Read the model definition and answer for the solid it produces. Units are mm, in the model's axes. A direction names the side the tool comes from. Give positions to 0.01 mm unless a question says otherwise; leave off trailing zeros. Loops run counter-clockwise (first coordinate to the right, second up) from the corner with the lowest first, then second, coordinate; pieces in that order, holes last. Notation, with made-up numbers: (38, 87) -> (94, 87) arc R13 cw to (94, 103) -> close; hole circle Ø11 at (-29.5, 3). An arc over 180 degrees is marked (long way). Return JSON: item names as keys, results as strings. Group by question number.
Autodesk Inventor part; units mm, degrees
ref_plane "YZ Plane" through (0, 0, 0) normal (1, 0, 0) x (0, 1, 0)
ref_plane "XZ Plane" through (0, 0, 0) normal (0, 1, 0) x (-1, 0, 0)
ref_plane "XY Plane" through (0, 0, 0) normal (0, 0, 1) x (1, 0, 0)
sketch "Sketch1" plane through (0, 0, 0) normal (1, 0, 0) x (0, 1, 0)
  arc A0 (-4.3875, 5.1282) -> (-5.1282, 4.3875) centre (0, 0) ccw
  arc A1 (-5.1895, 7.3532) -> (-4.3875, 5.1282) centre (-1.9912, 7.249) ccw
  arc A2 (-3.0589, 6.016) -> (-4.8075, 7.6084) centre (-5.9352, 4.6137) ccw
  arc A3 (-4.8075, 7.6084) -> (-5.1895, 7.3532) centre (0, 0) ccw
  arc A4 (-2.091, 6.4169) -> (-3.0589, 6.016) centre (0, 0) ccw
  arc A5 (-1.9805, 8.7794) -> (-2.091, 6.4169) centre (0.9345, 7.4592) ccw
  arc A6 (-1.5299, 8.869) -> (-1.9805, 8.7794) centre (0, 0) ccw
  arc A7 (-0.5238, 6.7286) -> (-1.5299, 8.869) centre (-3.7179, 6.5338) ccw
  arc A8 (0.5238, 6.7286) -> (-0.5238, 6.7286) centre (0, 0) ccw
  arc A9 (1.5299, 8.869) -> (0.5238, 6.7286) centre (3.7179, 6.5338) ccw
  arc A10 (1.9805, 8.7794) -> (1.5299, 8.869) centre (0, 0) ccw
  arc A11 (2.091, 6.4169) -> (1.9805, 8.7794) centre (-0.9345, 7.4592) ccw
  arc A12 (3.0589, 6.016) -> (2.091, 6.4169) centre (0, 0) ccw
  arc A13 (4.8075, 7.6084) -> (3.0589, 6.016) centre (5.9352, 4.6137) ccw
  arc A14 (5.1895, 7.3532) -> (4.8075, 7.6084) centre (0, 0) ccw
  arc A15 (4.3875, 5.1282) -> (5.1895, 7.3532) centre (1.9912, 7.249) ccw
  arc A16 (5.1282, 4.3875) -> (4.3875, 5.1282) centre (0, 0) ccw
  arc A17 (7.3532, 5.1895) -> (5.1282, 4.3875) centre (7.249, 1.9912) ccw
  arc A18 (7.6084, 4.8075) -> (7.3532, 5.1895) centre (0, 0) ccw
  arc A19 (6.016, 3.0589) -> (7.6084, 4.8075) centre (4.6137, 5.9352) ccw
  arc A20 (6.4169, 2.091) -> (6.016, 3.0589) centre (0, 0) ccw
  arc A21 (8.7794, 1.9805) -> (6.4169, 2.091) centre (7.4592, -0.9345) ccw
  arc A22 (8.869, 1.5299) -> (8.7794, 1.9805) centre (0, 0) ccw
  arc A23 (6.7286, 0.5238) -> (8.869, 1.5299) centre (6.5338, 3.7179) ccw
  arc A24 (6.7286, -0.5238) -> (6.7286, 0.5238) centre (0, 0) ccw
  arc A25 (8.869, -1.5299) -> (6.7286, -0.5238) centre (6.5338, -3.7179) ccw
  arc A26 (8.7794, -1.9805) -> (8.869, -1.5299) centre (0, 0) ccw
  arc A27 (6.4169, -2.091) -> (8.7794, -1.9805) centre (7.4592, 0.9345) ccw
  arc A28 (6.016, -3.0589) -> (6.4169, -2.091) centre (0, 0) ccw
  arc A29 (7.6084, -4.8075) -> (6.016, -3.0589) centre (4.6137, -5.9352) ccw
  arc A30 (7.3532, -5.1895) -> (7.6084, -4.8075) centre (0, 0) ccw
  arc A31 (5.1282, -4.3875) -> (7.3532, -5.1895) centre (7.249, -1.9912) ccw
  arc A32 (4.3875, -5.1282) -> (5.1282, -4.3875) centre (0, 0) ccw
  arc A33 (5.1895, -7.3532) -> (4.3875, -5.1282) centre (1.9912, -7.249) ccw
  arc A34 (4.8075, -7.6084) -> (5.1895, -7.3532) centre (0, 0) ccw
  arc A35 (3.0589, -6.016) -> (4.8075, -7.6084) centre (5.9352, -4.6137) ccw
  arc A36 (-8.869, 1.5299) -> (-6.7286, 0.5238) centre (-6.5338, 3.7179) ccw
  arc A37 (-6.7286, 0.5238) -> (-6.7286, -0.5238) centre (0, 0) ccw
  arc A38 (-6.7286, -0.5238) -> (-8.869, -1.5299) centre (-6.5338, -3.7179) ccw
  arc A39 (-8.869, -1.5299) -> (-8.7794, -1.9805) centre (0, 0) ccw
  arc A40 (-8.7794, -1.9805) -> (-6.4169, -2.091) centre (-7.4592, 0.9345) ccw
  arc A41 (-6.4169, -2.091) -> (-6.016, -3.0589) centre (0, 0) ccw
  arc A42 (-6.016, -3.0589) -> (-7.6084, -4.8075) centre (-4.6137, -5.9352) ccw
  arc A43 (-7.6084, -4.8075) -> (-7.3532, -5.1895) centre (0, 0) ccw
  arc A44 (-7.3532, -5.1895) -> (-5.1282, -4.3875) centre (-7.249, -1.9912) ccw
  arc A45 (-5.1282, -4.3875) -> (-4.3875, -5.1282) centre (0, 0) ccw
  arc A46 (-4.3875, -5.1282) -> (-5.1895, -7.3532) centre (-1.9912, -7.249) ccw
  arc A47 (-5.1895, -7.3532) -> (-4.8075, -7.6084) centre (0, 0) ccw
  arc A48 (-4.8075, -7.6084) -> (-3.0589, -6.016) centre (-5.9352, -4.6137) ccw
  arc A49 (-3.0589, -6.016) -> (-2.091, -6.4169) centre (0, 0) ccw
  arc A50 (-2.091, -6.4169) -> (-1.9805, -8.7794) centre (0.9345, -7.4592) ccw
  arc A51 (-1.9805, -8.7794) -> (-1.5299, -8.869) centre (0, 0) ccw
  arc A52 (-1.5299, -8.869) -> (-0.5238, -6.7286) centre (-3.7179, -6.5338) ccw
  arc A53 (-0.5238, -6.7286) -> (0.5238, -6.7286) centre (0, 0) ccw
  arc A54 (0.5238, -6.7286) -> (1.5299, -8.869) centre (3.7179, -6.5338) ccw
  arc A55 (1.5299, -8.869) -> (1.9805, -8.7794) centre (0, 0) ccw
  arc A56 (1.9805, -8.7794) -> (2.091, -6.4169) centre (-0.9345, -7.4592) ccw
  arc A57 (2.091, -6.4169) -> (3.0589, -6.016) centre (0, 0) ccw
  arc A58 (3.0589, -6.016) -> (4.8075, -7.6084) centre (5.9352, -4.6137) ccw
  arc A59 (4.8075, -7.6084) -> (5.1895, -7.3532) centre (0, 0) ccw
  arc A60 (5.1895, -7.3532) -> (4.3875, -5.1282) centre (1.9912, -7.249) ccw
  arc A61 (4.3875, -5.1282) -> (5.1282, -4.3875) centre (0, 0) ccw
  arc A62 (5.1282, -4.3875) -> (7.3532, -5.1895) centre (7.249, -1.9912) ccw
  arc A63 (7.3532, -5.1895) -> (7.6084, -4.8075) centre (0, 0) ccw
  arc A64 (7.6084, -4.8075) -> (6.016, -3.0589) centre (4.6137, -5.9352) ccw
  arc A65 (6.016, -3.0589) -> (6.4169, -2.091) centre (0, 0) ccw
  arc A66 (6.4169, -2.091) -> (8.7794, -1.9805) centre (7.4592, 0.9345) ccw
  arc A67 (8.7794, -1.9805) -> (8.869, -1.5299) centre (0, 0) ccw
  arc A68 (8.869, -1.5299) -> (6.7286, -0.5238) centre (6.5338, -3.7179) ccw
  arc A69 (6.7286, -0.5238) -> (6.7286, 0.5238) centre (0, 0) ccw
  arc A70 (6.7286, 0.5238) -> (8.869, 1.5299) centre (6.5338, 3.7179) ccw
  arc A71 (8.869, 1.5299) -> (8.7794, 1.9805) centre (0, 0) ccw
  arc A72 (8.7794, 1.9805) -> (6.4169, 2.091) centre (7.4592, -0.9345) ccw
  arc A73 (6.4169, 2.091) -> (6.016, 3.0589) centre (0, 0) ccw
  arc A74 (6.016, 3.0589) -> (7.6084, 4.8075) centre (4.6137, 5.9352) ccw
  arc A75 (7.6084, 4.8075) -> (7.3532, 5.1895) centre (0, 0) ccw
  arc A76 (7.3532, 5.1895) -> (5.1282, 4.3875) centre (7.249, 1.9912) ccw
  arc A77 (5.1282, 4.3875) -> (4.3875, 5.1282) centre (0, 0) ccw
  arc A78 (4.3875, 5.1282) -> (5.1895, 7.3532) centre (1.9912, 7.249) ccw
  arc A79 (5.1895, 7.3532) -> (4.8075, 7.6084) centre (0, 0) ccw
  arc A80 (4.8075, 7.6084) -> (3.0589, 6.016) centre (5.9352, 4.6137) ccw
  arc A81 (3.0589, 6.016) -> (2.091, 6.4169) centre (0, 0) ccw
  arc A82 (2.091, 6.4169) -> (1.9805, 8.7794) centre (-0.9345, 7.4592) ccw
  arc A83 (1.9805, 8.7794) -> (1.5299, 8.869) centre (0, 0) ccw
  arc A84 (1.5299, 8.869) -> (0.5238, 6.7286) centre (3.7179, 6.5338) ccw
  arc A85 (0.5238, 6.7286) -> (-0.5238, 6.7286) centre (0, 0) ccw
  arc A86 (-0.5238, 6.7286) -> (-1.5299, 8.869) centre (-3.7179, 6.5338) ccw
  arc A87 (-1.5299, 8.869) -> (-1.9805, 8.7794) centre (0, 0) ccw
  arc A88 (-1.9805, 8.7794) -> (-2.091, 6.4169) centre (0.9345, 7.4592) ccw
  arc A89 (-2.091, 6.4169) -> (-3.0589, 6.016) centre (0, 0) ccw
  arc A90 (-3.0589, 6.016) -> (-4.8075, 7.6084) centre (-5.9352, 4.6137) ccw
  arc A91 (-4.8075, 7.6084) -> (-5.1895, 7.3532) centre (0, 0) ccw
  arc A92 (-5.1895, 7.3532) -> (-4.3875, 5.1282) centre (-1.9912, 7.249) ccw
  arc A93 (-4.3875, 5.1282) -> (-5.1282, 4.3875) centre (0, 0) ccw
  arc A94 (-5.1282, 4.3875) -> (-7.3532, 5.1895) centre (-7.249, 1.9912) ccw
  arc A95 (-7.3532, 5.1895) -> (-7.6084, 4.8075) centre (0, 0) ccw
  arc A96 (-7.6084, 4.8075) -> (-6.016, 3.0589) centre (-4.6137, 5.9352) ccw
  arc A97 (-6.016, 3.0589) -> (-6.4169, 2.091) centre (0, 0) ccw
  arc A98 (-6.4169, 2.091) -> (-8.7794, 1.9805) centre (-7.4592, -0.9345) ccw
  arc A99 (-8.7794, 1.9805) -> (-8.869, 1.5299) centre (0, 0) ccw
  circle A100 centre (0, 0) radius 2.175
  line L0 (0, 0) -> (2.175, 0)
  line L1 (2.175, 0) -> (2.175, -1.2557)
  line L2 (2.175, -1.2557) -> (0, -2.5115)
  line L3 (-1.5245, 0) -> (0, 0)
  line L4 (0, 0) -> (0, -2.5115)
  line L5 (-2.175, 0) -> (-2.175, -1.2557)
  line L6 (-2.175, -1.2557) -> (0, -2.5115)
  line L7 (2.175, 0) -> (2.175, 1.2557)
  line L8 (2.175, 1.2557) -> (0, 2.5115)
  line L9 (-2.175, 0) -> (-2.175, 1.2557)
  line L10 (-2.175, 1.2557) -> (0, 2.5115)
  point P0 (0, -0.8741)
  point P1 (3.0589, -6.016)
  point P2 (-5.1282, 4.3875)
  point P3 (1.0875, -1.8836)
  point P4 (2.175, -0.6279)
  dimension "d14" = 120
  dimension "d17" = 4.35
extrude "Extrusion1" add sketch "Sketch1" along normal blind 3
equation "\"d17\" = d_agu"
equation "\"d_agu\" = 4.35"
properties part number "EngraneMod_v2"
1. Section A-A on y = 7 is taken. Determine the outline of the cut face in (x, z), then the cut area to 3 significant figures.
2. Section B-B on z = 5.5 is taken. Determine the outline of the cut face in (x, y).
3. Determine the mould class of faces 1 (the cylindrical face through (1.479, -0.815, -7.88)), 2 (the cylindrical face through (1.479, 0.815, 7.88)), 3 (the cylindrical face through (1.48, -2.26, -7.63)) for opening direction Z: pulls with the +Z half, pulls with the -Z half, needs draft (parallel to the pull), parting line crosses it, or undercut.
4. Straight lines are drawn through the part: line 1 (Y direction, x = 1.2, z = 0.25) (3 decimals); line 2 (Z direction, x = 1.15, y = 6.5); line 3 (Z direction, x = 0.45, y = 4.75). For each, find the intervals that lie inside material, in ascending order. Write a range as from..to.
5. Section C-C on y = 2.5 is taken. Determine the outline of the cut face in (x, z).
6. Which of the six approach directions +Z, -Z, +X, -X, +Y, -Y give full straight-line access (tool end or side, diameter ignored) to faces 4 (the flat face through (1, -2.175, 0)), 5 (the cylindrical face through (1.479, -7.88, 0.815)), 6 (the cylindrical face through (1.48, -0.83, 7.91)), 7 (the cylindrical face through (1.48, 6.99, 3.79))?
Completed:
{
 "1": {"outline": "(0, -5.18) -> (3, -5.18) -> (3, -3.8) -> (0, -3.8) -> close; (0, -2.23) -> (3, -2.23) -> (3, -0.55) -> (0, -0.55) -> close; (0, 0.55) -> (3, 0.55) -> (3, 2.23) -> (0, 2.23) -> close; (0, 3.8) -> (3, 3.8) -> (3, 5.18) -> (0, 5.18) -> close", "area": "18.4 mm²"},
 "2": {"outline": "(0, -4.67) -> (3, -4.67) -> (3, 4.67) -> (0, 4.67) -> close"},
 "3": {"face 1": "pulls with the -Z half", "face 2": "pulls with the +Z half", "face 3": "undercut"},
 "4": {"line 1": "y = -6.744..-2.175, 2.175..6.744", "line 2": "z = -5.1..-3.35, -2.12..2.12, 3.35..5.1", "line 3": "z = -7.59..-5.63, -4.79..4.79, 5.63..7.59"},
 "5": {"outline": "(0, -6.27) -> (3, -6.27) -> (3, 6.27) -> (0, 6.27) -> close"},
 "6": {"face 4": "+X, -X", "face 5": "+X, -X, -Y", "face 6": "+Z, +X, -X", "face 7": "+X, -X, +Y"}
}
